Here's how the part is built. I have some questions about the finished solid (model axes, mm). A direction names the side the tool comes from. Give positions to 0.01 mm unless a question says otherwise; leave off trailing zeros. Write each loop counter-clockwise with the first axis right and the second up, starting at its lowest first coordinate (ties: lowest second). Pieces come first, ordered by that corner, then holes. Notation, with made-up numbers: (-2, 76.5) -> (17, 76.5) arc R29 ccw to (17, 105.5) -> close; hole circle Ø4 at (5.5, 23). An arc over 180 degrees is marked (long way). Return JSON: item names as keys, results as strings.
from build123d import *

# Parameters (mm, degrees)
F0_W        = 15
F0_H        = 5
F1_DEPTH    = 38
F2_W        = 15
F2_H        = 5
F3_DEPTH    = 7
F4_T1_DEPTH = 50.0054850444
F1_FACE1_W  = 15
F1_FACE1_H  = 5
F8_DEPTH    = 15


# Not quite as in the source:
# - a fillet or chamfer that OpenCascade refuses, or shapes differently, is made with other operations: its cross-section is extruded or revolved along the edge and cut away or added


with BuildPart() as f1:
    # F0 (on Top) → F1 (new body)
    with BuildSketch(Plane.XY):
        with Locations((0, 2.5)):
            Rectangle(F0_W, F0_H)
    extrude(amount=F1_DEPTH)

    # F2 (on face) → F3 (join)
    with BuildSketch(Plane(origin=(0, 0, 0), x_dir=(1, 0, 0), z_dir=(0, 0, -1))):
        Polygon((7.5, -10), (7.5, -5), (-7.5, -5), (-7.5, -10), (-7.5, -11), (0, -12.5), (7.5, -11), align=None)
        with Locations((0, -2.5)):
            Rectangle(F2_W, F2_H)
    extrude(amount=F3_DEPTH)

    # F4: chamfer of 2.5 x 7.5152772587 on 2 edges, made by hand

    # F4_s2 → F4_t1 (cut)
    with BuildSketch(Plane.XZ.offset(-30.5027425222)):
        Polygon((0.0152772587, -7), (-7.5, -4.5), (-7.5, -7), align=None)
        Polygon((-0.0152772587, -7), (7.5, -4.5), (7.5, -7), align=None)
    extrude(amount=F4_T1_DEPTH, mode=Mode.SUBTRACT)

    # F6: sweep along a path in F5
    with BuildLine(Plane.YZ.offset(7.5)) as f6_path:
        ThreePointArc((17.5, 38), (10, 45.5), (2.5, 38))
    # F1_face1 (on face) → F6 (sweep)
    with BuildSketch(Plane(origin=(0, 2.5, 38), x_dir=(1, 0, 0), z_dir=(0, 0, 1))):
        Rectangle(F1_FACE1_W, F1_FACE1_H)
    sweep(path=f6_path.line)

    # F7 (on face) → F8 (join)
    with BuildSketch(Plane.YZ.offset(7.5)):
        Polygon((6, 30), (5, 38), (5, 30), align=None)
    extrude(amount=-F8_DEPTH)


solid = f1.part
1. Suppose I cut it at D-D, the plane y = 3.75. List the corners of the cut face in (x, z) for me.
Taken from the geometry:
{"outline": "(-7.5, -4.5) -> (0, -6.99) -> (7.5, -4.5) -> (7.5, 45.81) -> (-7.5, 45.81) -> close"}
2. If I drill on line 1 (Z direction, x = -1, y = 10); line 2 (Y direction, x = -4.5, z = 6.5); line 3 (Z direction, x = 3, y = 6.5), over which ranges is the centre line in solid material (lowest first)? Write a range as [from, to].
Taken from the geometry:
{"line 1": "z = [-6.66, 0], [43, 48]", "line 2": "y = [0, 5]", "line 3": "z = [-6, 0], [41.57, 47.37]"}
3. Which directions (+Z, -Z, +X, -X, +Y, -Y) give clear straight access to the entire face, cutting with the end or side of a thin tool? Please do faces 4 (the face through (0, 18, 38)), 5 (the face through (-3.8, 11.74, -2.67)), 6 (the face through (0, 9, 0)), 7 (the face through (0, 0, 16)).
Taken from the geometry:
{"face 4": "-Z, +X, -X, +Y", "face 5": "-Z, -X, +Y", "face 6": "+X, -X, +Y", "face 7": "+Z, -Z, +X, -X, -Y"}
4. Suppose I cut it at B-B, the plane x = 4.5. List the corners of the cut face in (y, z) for me.
Taken from the geometry:
{"outline": "(0, -5.5) -> (11.6, -5.5) -> (11.6, 0) -> (5, 0) -> (5, 30) -> (6, 30) -> (5, 38) arc R5 cw to (15, 38) -> (20, 38) arc R10 ccw to (0, 38) -> close"}
5. Suppose I cut it at C-C, the plane z = 27. List the corners of the cut face in (x, y) for me.
Taken from the geometry:
{"outline": "(-7.5, 0) -> (7.5, 0) -> (7.5, 5) -> (-7.5, 5) -> close"}
6. Suppose I cut it at A-A, the plane y = 10. List the corners of the cut face in (x, z) for me, and give its area (3 significant figures).
Taken from the geometry:
{"outline": "(-7.5, -4.5) -> (0, -6.99) -> (7.5, -4.5) -> (7.5, 0) -> (-7.5, 0) -> close; (-7.5, 43) -> (7.5, 43) -> (7.5, 48) -> (-7.5, 48) -> close", "area": "161 mm²"}
7. If we mould it in two halves opening along Y, with no side actions, what happens to faces 1 (the face through (3.7, 11.76, -2.67)), 2 (the face through (0, 10, 43)), 3 (the face through (0.1, 5.5, 30))? For each: released by +Y, released by -Y, zero draft, split by the parting line, or undercut.
Taken from the geometry:
{"face 1": "released by +Y", "face 2": "undercut", "face 3": "zero draft"}
8. For pin 1 Ø8 at (x, z) = (-5, 33) entering from +Y; pin 2 Ø8 at (y, z) = (8.5, 3) entering from -X; pin 3 Ø1.5 at (x, z) = (-3.5, 12.5) entering from +Y; pin 4 Ø2 at (x, y) = (-6, 6.5) entering from -Z, each with a flat end and sliding along its axis, tell me the tip position at first contact or that it passes through.
Taken from the geometry:
{"pin 1": "stops at y = 6", "pin 2": "stops at x = -7.5", "pin 3": "stops at y = 5", "pin 4": "stops at z = -5.33"}
